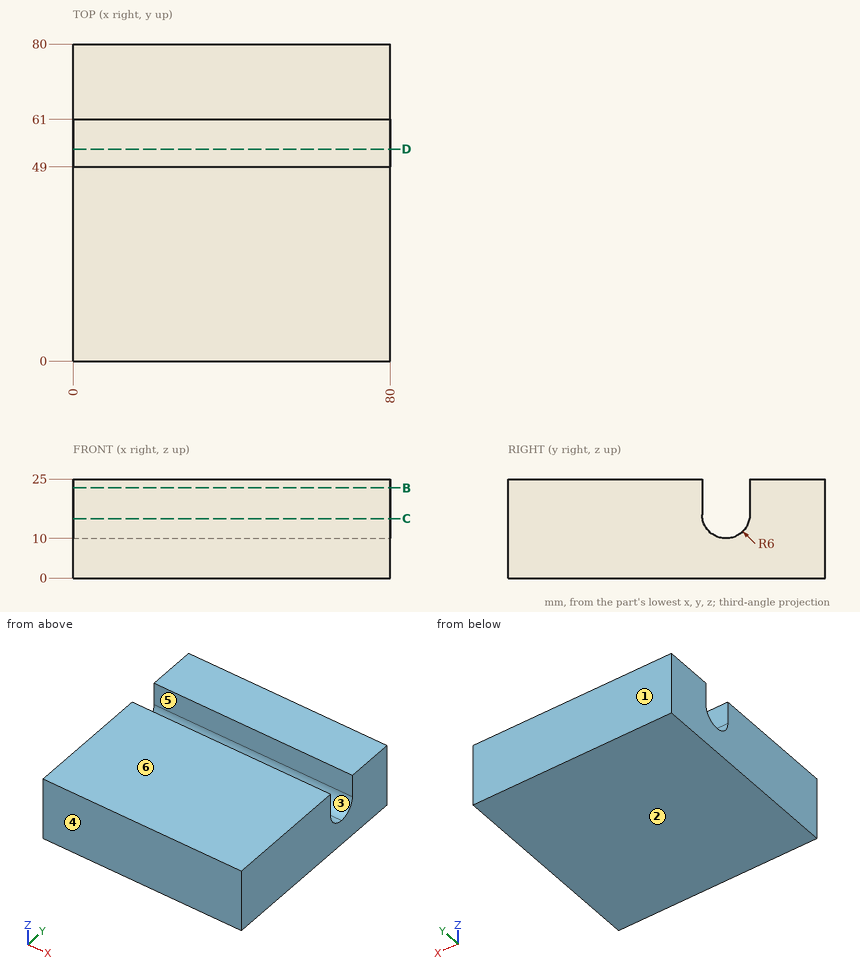
Geometry check sheet. Reference: drawing and pictorial views, mm from the part's lowest x, y, z. A direction names the side the tool comes from. Round coordinates to 2 decimals unless told otherwise and drop trailing zeros. Loops run counter-clockwise (first coordinate to the right, second up) from the corner with the lowest first, then second, coordinate; pieces in that order, holes last. Notation, with made-up numbers: (-30.75, 72.25) - (-9.75, 72.25) arc R16 ccw to (-9.75, 77.25) - close; hole circle Ø2 at (1, -14.5). An arc over 180 degrees is marked (long way). One line per question, with ' | ' between items. Start each with the question number.
1. Cross-section at C-C on z = 15. Record the cut outline in (x, y), then the cut area to 3 significant figures.
2. Cross-section at D-D on y = 53.5. Record the cut outline in (x, z), then the cut area to 3 significant figures.
3. Draft check along Y on the marked faces 1, 2, 3 and 4. Enter one of: released by +Y, released by -Y, zero draft, split by the parting line, or undercut.
4. Cross-section at B-B on z = 22.75. Record the cut outline in (x, y), then the cut area to 3 significant figures.
5. Tool access check on the marked faces 5 and 6. Record the directions out of +Z, -Z, +X, -X, +Y, -Y that give a thin tool (end or side, any length) a straight path to the whole face; none if there is none.
6. Scan lines: line 1 (Y direction, x = 19.5, z = 23); line 2 (Y direction, x = 27, z = 11). Record each from-to range of solid material in increasing order. Write a range as [from, to].
Taken from the geometry:
1) outline: (0, 0) - (80, 0) - (80, 49.08) - (0, 49.08) - close; (0, 60.92) - (80, 60.92) - (80, 80) - (0, 80) - close | area: 5,450 mm²
2) outline: (0, 0) - (80, 0) - (80, 10.19) - (0, 10.19) - close | area: 815 mm²
3) face 1: released by +Y | face 2: zero draft | face 3: undercut | face 4: released by -Y
4) outline: (0, 0) - (80, 0) - (80, 49) - (0, 49) - close; (0, 61) - (80, 61) - (80, 80) - (0, 80) - close | area: 5,440 mm²
5) face 5: +Z, +X, -X | face 6: +Z, +X, -X, +Y, -Y
6) line 1: [0, 49], [61, 80] | line 2: [0, 51.68], [58.32, 80]
